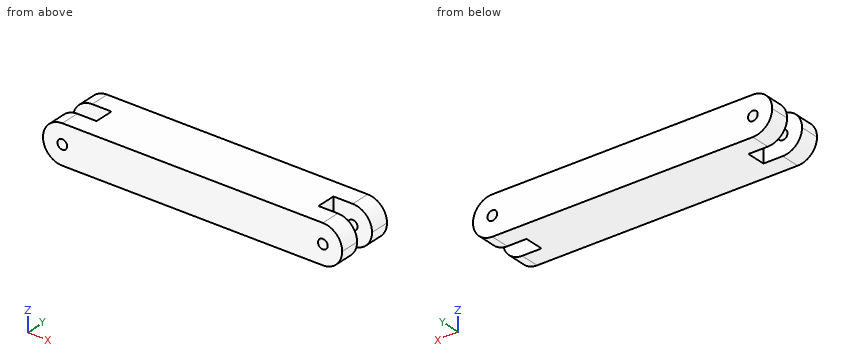
Solid Edge part; units mm, degrees
sketch "Sketch1" plane through (0, 0, 0) normal (0, 0, 1) x (1, 0, 0)
  line L0 (57.5, -5) -> (77.5, -5)
  line L1 (77.5, -5) -> (77.5, -15)
  line L2 (77.5, -15) -> (-77.5, -15)
  line L3 (-77.5, -15) -> (-77.5, -5)
  line L4 (-57.5, -5) -> (-77.5, -5)
  line L5 (-57.5, 5) -> (-57.5, -5)
  line L6 (-77.5, 5) -> (-57.5, 5)
  line L7 (-77.5, 5) -> (-77.5, 15)
  line L8 (-77.5, 15) -> (77.5, 15)
  line L9 (77.5, 15) -> (77.5, 5)
  line L10 (77.5, 5) -> (57.5, 5)
  line L11 (57.5, 5) -> (57.5, -5)
extrude "Protrusion1" add sketch "Sketch1" along normal blind 20
sketch "Sketch2" plane through (0, -15, 10) normal (0, -1, 0) x (1, 0, 0)
  circle A0 centre (67.5, 0) radius 2.5
  circle A1 centre (-67.5, 0) radius 2.5
extrude "Cutout1" cut sketch "Sketch2" against normal up to surface (30 mm away)
fillet "Redondeo_1" radius 10 8 edges at (77.5, -10, 20) (77.5, 10, 20) (77.5, -10, 0) (77.5, 10, 0) (-77.5, 10, 20) (-77.5, -10, 20) (-77.5, -10, 0) (-77.5, 10, 0)
Could you check a few things on this model? Use its own coordinates, in mm. Coordinates: 2 decimals unless noted, no trailing zeros. Order: outer loops, then holes, each group sorted by start corner. A loop starts at its lowest first (then second) coordinate and runs counter-clockwise, first axis right, second up. Notation, with made-up numbers: M -31,28.25 L 1,28.25 A31 cw 1,57.25 Z; hole C -32,73.5 d10. An arc over 180 degrees is marked long. Use one line per item in the form item = value. Start each with the question number.
1. Suppose I cut it at B-B on y = 11. Count the separate pieces of the cut face and the enclosed holes in it, then the cut area to 3 significant figures.
2. Suppose I cut it at A-A on x = 61.5. Write out the boundary of the cut face in (y, z).
3. Please list where these lines run through material, in increasing order: line 1 (Y direction, x = 58, z = 11.5); line 2 (Z direction, x = 67.5, y = 8.5); line 3 (X direction, y = 9, z = 10.5).
4. Suppose I cut it at C-C on z = 1.5. Write out the boundary of the cut face in (x, y), then the cut area to 3 significant figures.
5. Suppose I cut it at D-D on y = 3.5. Write out the boundary of the cut face in (x, z), then the cut area to 3 significant figures.
6. For pin 1 (8 mm diameter, centred on x = 67.5, z = 10, fed in from -Y); pin 2 (1 mm diameter, centred on y = 5, z = 12.5, fed in from -X); pin 3 (8 mm diameter, centred on y = -5.5, z = 2.5, fed in from +X); pin 4 (8 mm diameter, centred on y = 0.5, z = 11, fed in from -X), each with a flat end and sliding along its axis, tell me the tip position at first contact or that it passes through.
Geometry says:
q1.separate_pieces = 1
q1.enclosed_holes = 2
q1.area = 2,970 mm^2
q2.outline = M -15,0 L -5,0 L -5,20 L -15,20 Z; M 5,0 L 15,0 L 15,20 L 5,20 Z
q3.line_1 = -15 to -5, 5 to 15
q3.line_2 = 0 to 7.5, 12.5 to 20
q3.line_3 = -77.49 to -69.95, -65.05 to 65.05, 69.95 to 77.49
q4.outline = M -72.77,-15 L 72.77,-15 L 72.77,-5 L 57.5,-5 L 57.5,5 L 72.77,5 L 72.77,15 L -72.77,15 L -72.77,5 L -57.5,5 L -57.5,-5 L -72.77,-5 Z
q4.area = 4,060 mm^2
q5.outline = M -57.5,0 L 57.5,0 L 57.5,20 L -57.5,20 Z
q5.area = 2,300 mm^2
q6.pin_1 = -15
q6.pin_2 = -77.3
q6.pin_3 = 76.87
q6.pin_4 = -57.5
